Geometry: final body of the model. Coordinates: model frame, mm. Face numbers are marked on the shaded views. A direction names the side the tool comes from. Give positions to 0.01 mm unless a question says otherwise; leave off trailing zeros. Loops run counter-clockwise (first coordinate to the right, second up) from the corner with the lowest first, then second, coordinate; pieces in that order, holes last. Notation, with made-up numbers: (-17.75, -23) -> (-13.75, -23) arc R11 cw to (-13.75, -10) -> close; hole circle Ø6 at (0, -11). An arc over 180 degrees is marked (long way). One line per question, with ' | ' between items. Start each with the question number.
Item 1: Pin query (flat end, axial travel): P1, Ø2.5, axis at x = 0, y = 4, coming from the +Z side; P2, Ø3, axis at x = -8, y = 5, coming from the +Z side; P3, Ø3, axis at y = 1, z = 6.5, coming from the -X side. Return the tip coordinate at first contact, or that it passes through.
Item 2: Section D-D on x = 6. Return loops of the section in (y, z).
Item 3: Section A-A on x = -1. Return loops of the section in (y, z), then the cut area to 3 significant figures.
Item 4: Set-up query: the marked faces 1 and 2. Return all of +Z, -Z, +X, -X, +Y, -Y with unobstructed straight access to the full face (end or side cutting, diameter ignored); none if empty.
Item 5: Section B-B on y = 4.7. Return loops of the section in (x, z).
Item 6: Mould query, pull axis Z, two halves, no side actions, for the marked faces 3, 4 and 5. Classes: released by +Z, released by -Z, zero draft, split by the parting line, or undercut.
Item 7: Section C-C on z = 6.5. Return loops of the section in (x, y), then the cut area to 3 significant figures.
Item 8: Material intervals for line 1 along Z through (x, y) = (-1, 4.95); line 2 along Y through (x, z) = (2, 10); line 3 along X through (y, z) = (2.95, 1.75), sorted ascending. Write a range as [from, to].
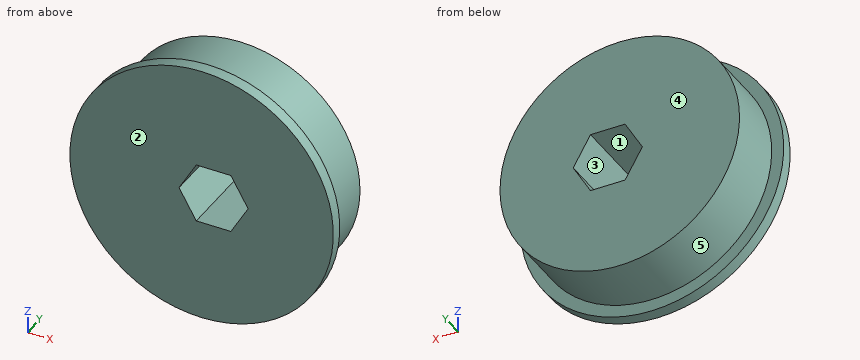
from build123d import *

# Parameters (mm, degrees)
SKETCH1_R           = 10
BOSS_EXTRUDE1_DEPTH = 6
SKETCH2_R           = 11
BOSS_EXTRUDE2_DEPTH = 1
CUT_EXTRUDE1_DEPTH  = 18.349351573


with BuildPart() as part:
    # Sketch1 → Boss-Extrude1 (new body)
    with BuildSketch(Plane(origin=(0, 0, 0), x_dir=(1, 0, 0), z_dir=(0, 1, 0))):
        with Locations(Location((-1, 0, 0), (0, 0, 270))):
            Circle(SKETCH1_R)
    extrude(amount=BOSS_EXTRUDE1_DEPTH)

    # Sketch2 → Boss-Extrude2 (add)
    with BuildSketch(Plane.XZ):
        with Locations(Location((-1, 0, 0), (0, 0, 270))):
            Circle(SKETCH2_R)
    extrude(amount=-BOSS_EXTRUDE2_DEPTH)

    # Sketch4 → Cut-Extrude1 (cut, through all)
    with BuildSketch(Plane(origin=(0, 6, 0), x_dir=(1, 0, 0), z_dir=(0, 1, 0))):
        Polygon((2.886751346, 0), (1.443375673, 2.5), (-1.443375673, 2.5), (-2.886751346, 0), (-1.443375673, -2.5), (1.443375673, -2.5), align=None)
    extrude(amount=-CUT_EXTRUDE1_DEPTH, mode=Mode.SUBTRACT)


solid = part.part
Result sheet:
1) P1: stops at z = 10 | P2: stops at z = 8.35 | P3: stops at x = -10.8
2) outline: (0, -8.49) -> (1, -8.49) -> (1, -7.14) -> (6, -7.14) -> (6, 7.14) -> (1, 7.14) -> (1, 8.49) -> (0, 8.49) -> close
3) outline: (0, -11) -> (1, -11) -> (1, -10) -> (6, -10) -> (6, -2.5) -> (0, -2.5) -> close; (0, 2.5) -> (6, 2.5) -> (6, 10) -> (1, 10) -> (1, 11) -> (0, 11) -> close | area: 92.0 mm²
4) face 1: +Y, -Y | face 2: +Z, -Z, +X, -X, -Y
5) outline: circle Ø20 at (-1, 0); hole (-2.89, 0) -> (-1.44, -2.5) -> (1.44, -2.5) -> (2.89, 0) -> (1.44, 2.5) -> (-1.44, 2.5) -> close
6) face 3: undercut | face 4: zero draft | face 5: split by the parting line
7) outline: (-9.87, 0) -> (7.87, 0) -> (7.87, 1) -> (6.6, 1) -> (6.6, 6) -> (-8.6, 6) -> (-8.6, 1) -> (-9.87, 1) -> close | area: 93.7 mm²
8) line 1: z = [-10, -2.5], [2.5, 10] | line 2: y = [0, 1] | line 3: x = [-10.85, -1.88], [1.88, 8.85]
